Geometry check sheet. Reference: drawing and pictorial views, mm from the part's lowest x, y, z. A direction names the side the tool comes from. Give positions to 0.01 mm unless a question says otherwise; leave off trailing zeros. Loops run counter-clockwise (first coordinate to the right, second up) from the corner with the lowest first, then second, coordinate; pieces in that order, holes last. Notation, with made-up numbers: (88, 21) - (126, 21) arc R16 ccw to (126, 50) - close; hole circle Ø1 at (-0.5, 24). An arc over 180 degrees is marked (long way). Answer in a Markdown table with one row per item. Add a question column.
(1) Draft check along X on the marked faces 1, 2 and 3. Enter one of: released by +X, released by -X, zero draft, split by the parting line, or undercut.
(2) Thickness scan on L1, parallel to Y at x = 43, z = 2; L2, parallel to X at y = 12.25, z = 2.5; L3, parallel to X at y = 14.75, z = 3.5 (1 decimal). Record the ranges inside material, lowest first.
(3) Go/stop test with flat-tipped pins: P1, Ø1.5, axis at y = 11, z = 3, coming from the -X side; P2, Ø3, axis at x = 37, z = 6, coming from the -Y side. Record where each tip stops, or that it passes through.
(4) Set-up check for the marked faces 4 and 5: record each of +Z, -Z, +X, -X, +Y, -Y from which the full face is reachable in a straight line by a thin tool's end or side.
(5) Sectioned sample at C-C on y = 15.5. Enter the section's corners in (x, z) (1 decimal).
(6) Sectioned sample at A-A on x = 76. Enter the section's corners in (y, z).
(7) Sectioned sample at B-B on z = 7. Enter the section's corners in (x, y).
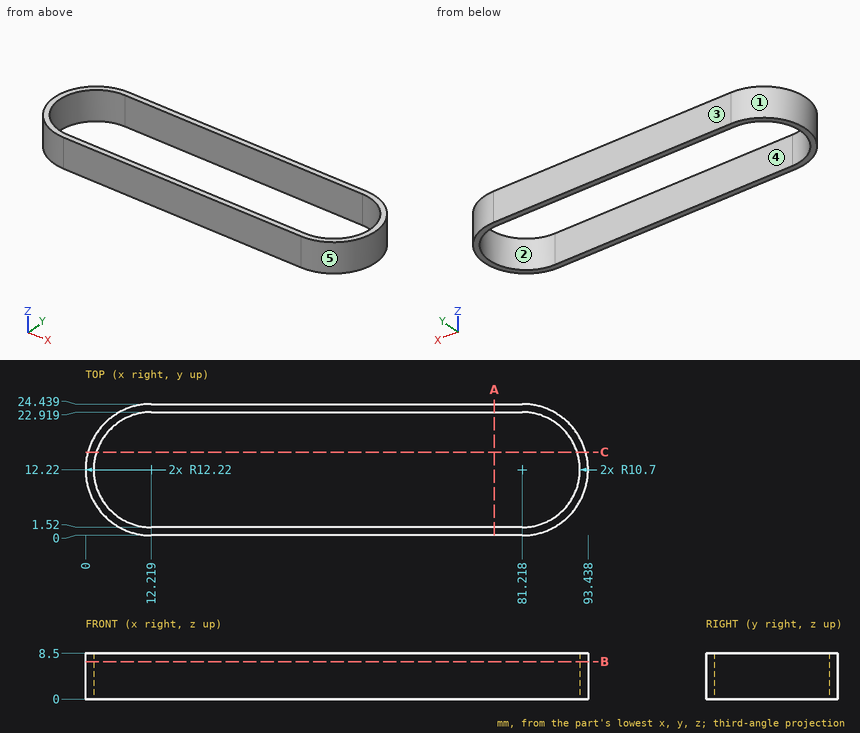
Reply:
| question | item | result |
|---|---|---|
| 1 | face 1 | released by -X |
| 1 | face 2 | undercut |
| 1 | face 3 | zero draft |
| 2 | L1 | 0 to 1.52, 22.92 to 24.44 |
| 2 | L2 | 0 to 1.52, 91.92 to 93.44 |
| 2 | L3 | 0.3 to 1.8, 91.6 to 93.2 |
| 3 | P1 | x = 0.01 |
| 3 | P2 | y = 0 |
| 4 | face 4 | +Z, -Z |
| 4 | face 5 | +Z, -Z, +X |
| 5 | outline | (0.4, 0) - (2, 0) - (2, 8.5) - (0.4, 8.5) - close; (91.4, 0) - (93, 0) - (93, 8.5) - (91.4, 8.5) - close |
| 6 | outline | (0, 0) - (1.52, 0) - (1.52, 8.5) - (0, 8.5) - close; (22.92, 0) - (24.44, 0) - (24.44, 8.5) - (22.92, 8.5) - close |
| 7 | outline | (12.22, 0) - (81.22, 0) arc R12.22 ccw to (81.22, 24.44) - (12.22, 24.44) arc R12.22 ccw to start; hole (12.22, 1.52) - (81.22, 1.52) arc R10.7 ccw to (81.22, 22.92) - (12.22, 22.92) arc R10.7 ccw to start |
